Could you check a few things on this model? Use its own coordinates, in mm. A direction names the side the tool comes from. Give positions to 0.01 mm unless a question says otherwise; leave off trailing zeros. Write each loop counter-clockwise with the first axis right and the second up, starting at its lowest first coordinate (ties: lowest second). Pieces come first, ordered by that corner, then holes. Notation, with made-up numbers: (-5, 38) - (41, 38) arc R20 ccw to (41, 72) - close; hole circle Ø11 at (43, 44). An arc over 180 degrees is marked (long way). Answer as CSV lines item,"result". Start each with the question number.
Q1. Imagine slicing it at C-C on z = -15.5. List the corners of the cut face in (x, y) for me.
Q2. Imagine slicing it at B-B on x = 0. List the corners of the cut face in (y, z) for me, and give its area (3 significant figures).
Q3. Will these pins go through, and if not, where does the flat tip stop? pin 1 Ø2 at (y, z) = (8, -10.5) entering from +X; pin 2 Ø1 at (x, z) = (15.5, -10) entering from +Y; pin 3 Ø11.5 at (y, z) = (0, -8) entering from +X; pin 4 Ø1.5 at (x, z) = (15, -0.5) entering from -Y.
Q4. We'd pull the mould along Z, two halves only. Please class faces 1 (the face through (-7.3, -22.1, 16)), 2 (the face through (7.509, 23.846, 13.014)), 3 (the face through (0, 0, 8)): pulls with the +Z half, pulls with the -Z half, needs draft (parallel to the pull), parting line crosses it, or undercut.
Q5. On a 3-axis mill with a long thin cutter (end or side, diameter ignored), from which of +Z, -Z, +X, -X, +Y, -Y can I reach the whole of each face in a straight line? I mean faces 4 (the face through (-23.73, -2.74, -3.7)), 5 (the face through (22.804, -2.994, 15.014)), 6 (the face through (22.453, -4.986, -6.311)). Say none if no direction works.
Q6. Imagine slicing it at A-A on z = -8. List the corners of the cut face in (x, y) for me, and give its area (3 significant figures).
Q7. If I drill on line 1 along Z through (x, y) = (24.4, 0); line 2 along Z through (x, y) = (9.5, 4); line 3 along Y through (x, z) = (-2.5, -15.5), over which ranges is the centre line in solid material (lowest first)?
Q8. Imagine slicing it at D-D on y = 0. State how many separate pieces and enclosed holes the cut face has, and give its area (3 significant figures).
```python
from build123d import *

# Parameters (mm, degrees)
F2_R = 2
F7_D = 10.2


with BuildPart() as f1:
    # F0 (on Right) → F1 (revolve)
    with BuildSketch(Plane.YZ):
        Polygon((25, 20), (0, 20), (0, 16), (0, -20), (25, -20), (25, 10), (23, 10), (23, 12), (25, 12), (25, 14), (23, 14), (23, 16), (25, 16), align=None)
    revolve(axis=Axis((0, 0, -4), (0, 0, -1)))

    # F2
    f2_edges = [f1.edges().sort_by_distance(p)[0] for p in [
        (0, -25, 20),
    ]]
    fillet(f2_edges, radius=F2_R)

    # F3 (on Right) → F4 (revolve, cut)
    with BuildSketch(Plane.YZ):
        with BuildLine():
            Line((0, 8), (0, -20))
            Line((0, -20), (23, -20))
            Line((23, -20), (23, 7))
            ThreePointArc((23, 7), (22.707107, 7.707107), (22, 8))
            Line((22, 8), (0, 8))
        make_face()
    revolve(axis=Axis((0, 0, -6), (0, 0, 1)), mode=Mode.SUBTRACT)

    # F7 (through all)
    with Locations(Plane.YZ.offset(25)):
        with Locations((0, -8)):
            Hole(F7_D / 2)


solid = f1.part
```
Conclusion:
1,outline,"circle Ø50 at (0, 0); hole circle Ø46 at (0, 0)"
2,outline,"(-25, -20) - (-23, -20) - (-23, 7) arc R1 cw to (-22, 8) - (22, 8) arc R1 cw to (23, 7) - (23, -20) - (25, -20) - (25, 10) - (23, 10) - (23, 12) - (25, 12) - (25, 14) - (23, 14) - (23, 16) - (25, 16) - (25, 18) arc R2 ccw to (23, 20) - (-23, 20) arc R2 ccw to (-25, 18) - (-25, 16) - (-23, 16) - (-23, 14) - (-25, 14) - (-25, 12) - (-23, 12) - (-23, 10) - (-25, 10) - close"
2,area,"695 mm^2"
3,pin 1,"x = 24"
3,pin 2,"y = 20"
3,pin 3,"x = 25"
3,pin 4,"y = -20.54"
4,face 1,"undercut"
4,face 2,"needs draft"
4,face 3,"pulls with the -Z half"
5,face 4,"+X, -X"
5,face 5,"none"
5,face 6,"-Z"
6,outline,"(-24.47, -5.1) arc R25 ccw to (24.47, -5.1) - (22.43, -5.1) arc R23 cw to (-22.43, -5.1) - close; (-24.47, 5.1) - (-22.43, 5.1) arc R23 cw to (22.43, 5.1) - (24.47, 5.1) arc R25 ccw to start"
6,area,"260 mm^2"
7,line 1,"-20 to -13.1, -2.9 to 10, 12 to 14, 16 to 19.43"
7,line 2,"8 to 20"
7,line 3,"-24.87 to -22.86, 22.86 to 24.87"
8,separate pieces,"3"
8,enclosed holes,"0"
8,area,"654 mm^2"
